Source: CAD feature listing. Evaluate the final solid. Frame: model axes, mm. Face numbers are marked on the shaded views. A direction names the side the tool comes from. Round coordinates to 2 decimals unless told otherwise and drop trailing zeros. Order: outer loops, then holes, each group sorted by start corner. A loop starts at its lowest first (then second) coordinate and runs counter-clockwise, first axis right, second up.
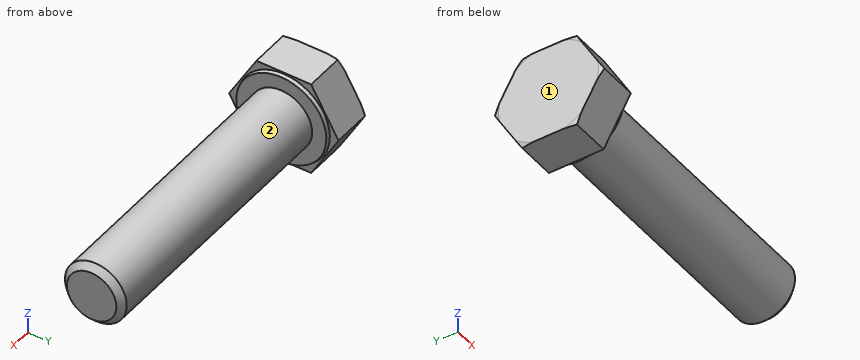
```python
from build123d import *

# Parameters (mm, degrees)
SKETCH_2_OUTSIDE_W  = 31.274
SKETCH_2_OUTSIDE_H  = 31.274
CUT_EXTRUDE_1_DEPTH = 54.660016772
CHAMFER_1_SIZE      = 1


with BuildPart() as part:
    # Эскиз1 → Повернуть1 (revolve)
    with BuildSketch(Plane.XY, mode=Mode.PRIVATE) as revolve_1_sk:
        Polygon((-6.58, 0), (-6.58, 8.85), (0, 8.85), (0, 7.448974596), (0.6, 7.288205081), (0.6, 5), (45.6, 5), (45.6, 0), align=None)
    revolve(revolve_1_sk.sketch.rotate(Axis((-1000, 0, 0), (1, 0, 0)), 90), axis=Axis((-1000, 0, 0), (1, 0, 0)))

    # Эскиз2 outside → Вырез-Вытянуть1 (cut, through all)
    with BuildSketch(Plane.ZY.offset(6.58)):
        Rectangle(SKETCH_2_OUTSIDE_W, SKETCH_2_OUTSIDE_H)
        Polygon((0, -8.85), (7.664324823, -4.425), (7.664324823, 4.425), (0, 8.85), (-7.664324823, 4.425), (-7.664324823, -4.425), align=None, mode=Mode.SUBTRACT)
    extrude(amount=-CUT_EXTRUDE_1_DEPTH, mode=Mode.SUBTRACT)

    # Эскиз4 → Вырез-Повернуть1 (revolve, cut)
    with BuildSketch(Plane.XY):
        Polygon((-6.58, 8.075), (-6.297923068, 8.85), (-6.58, 8.85), align=None)
    revolve(axis=Axis((-1000, 0, 0), (1, 0, 0)), mode=Mode.SUBTRACT)

    # Фаска1
    chamfer_1_edges = [part.edges().sort_by_distance(p)[0] for p in [
        (45.6, 0, -5),
    ]]
    chamfer(chamfer_1_edges, length=CHAMFER_1_SIZE)


solid = part.part
```
1. First-contact query: pin 1 (5 mm diameter, centred on x = 8, y = 0, fed in from +Z); pin 2 (2 mm diameter, centred on x = -1, y = -4.5, fed in from +Z); pin 3 (1.5 mm diameter, centred on y = -5.5, z = 1.5, fed in from +X); pin 4 (5 mm diameter, centred on x = 24, z = -6, fed in from +Y). Flat tips, straight axial feed; report the tip coordinate or a pass-through.
2. Line query: line 1 along Y through (x, z) = (31.5, -3); line 2 along X through (y, z) = (4.25, 5); line 3 along Y through (x, z) = (39.5, 0). Output: solid intervals per line, ascending.
3. Access query for the marked faces 1 and 2. Directions: +Z, -Z, +X, -X, +Y, -Y. A direction counts if a zero-diameter tool reaches every point of the face in a straight line with its end or side. Return the directions, or none.
4. Section C-C on x = 11. Return loops of the section in (y, z).
5. Section A-A on y = 0. Return loops of the section in (x, z), plus the area to 3 significant figures.
6. Section B-B on x = -2.5. Return loops of the section in (y, z) (3 decimals).
Result:
1. pin 1: stops at z = 5
1. pin 2: stops at z = 7.66
1. pin 3: stops at x = 44.65
1. pin 4: stops at y = 3.57
2. line 1: y = -4 to 4
2. line 2: x = -6.58 to 0.6
2. line 3: y = -5 to 5
3. face 1: +Z, -Z, -X, +Y, -Y
3. face 2: +X
4. outline: circle Ø10 at (0, 0)
5. outline: (-6.58, -7.66) - (0, -7.66) - (0, -7.45) - (0.6, -7.29) - (0.6, -5) - (44.6, -5) - (45.6, -4) - (45.6, 4) - (44.6, 5) - (0.6, 5) - (0.6, 7.29) - (0, 7.45) - (0, 7.66) - (-6.58, 7.66) - close
5. area: 559 mm2
6. outline: (-8.85, 0) - (-4.425, -7.664) - (4.425, -7.664) - (8.85, 0) - (4.425, 7.664) - (-4.425, 7.664) - close
